Read the model definition and answer for the solid it produces. Units are mm, in the model's axes. A direction names the side the tool comes from. Give positions to 0.01 mm unless a question says otherwise; leave off trailing zeros. Order: outer loops, then holes, each group sorted by start corner. A loop starts at its lowest first (then second) coordinate and runs counter-clockwise, first axis right, second up.
```python
from build123d import *

# Parameters (mm, degrees)
EXTRUDE_1_DEPTH = 3
CHAMFER_1_SIZE  = 0.3065
CHAMFER_2_SIZE  = 0.5
FILLET_1_R      = 0.3


with BuildPart() as part:
    # 草圖1 → 填料-伸長1 (new body)
    with BuildSketch(Plane(origin=(-3, 0, 0), x_dir=(0, -1, 0), z_dir=(-1, 0, 0))):
        with BuildLine():
            Line((2.449489743, 2.5), (-2.449489743, 2.5))
            ThreePointArc((-2.449489743, 2.5), (-3.5, 0), (-2.449489743, -2.5))
            Line((-2.449489743, -2.5), (2.449489743, -2.5))
            ThreePointArc((2.449489743, -2.5), (3.5, 0), (2.449489743, 2.5))
        make_face()
    extrude(amount=-EXTRUDE_1_DEPTH)

    # 草圖2 → 旋轉1 (revolve)
    with BuildSketch(Plane.XY, mode=Mode.PRIVATE) as revolve_1_sk:
        Polygon((0, 1.95), (0, 0), (11, 0), (11, 1.5), (6.2, 1.5), (6.2, 1.05), (5, 1.05), (5, 2), (1.5, 2), (1.5, 1.95), align=None)
    revolve(revolve_1_sk.sketch.rotate(Axis((0, 0, 0), (1, 0, 0)), 270), axis=Axis((0, 0, 0), (1, 0, 0)))

    # 導角1
    chamfer_1_edges = [part.edges().sort_by_distance(p)[0] for p in [
        (11, 0, 1.5),
    ]]
    chamfer(chamfer_1_edges, length=CHAMFER_1_SIZE)

    # 導角2
    chamfer_2_edges = [part.edges().sort_by_distance(p)[0] for p in [
        (-3, 3.5, 0),
        (-3, -3.5, 0),
    ]]
    chamfer(chamfer_2_edges, length=CHAMFER_2_SIZE)

    # 圓角1
    fillet_1_edges = [part.edges().sort_by_distance(p)[0] for p in [
        (6.2, 0, 1.05),
        (5, 0, 1.05),
    ]]
    fillet(fillet_1_edges, radius=FILLET_1_R)


solid = part.part
```
1) The part is cut by section A-A on z = 0. Determine the outline of the cut face in (x, y), and give its area (3 significant figures).
Final values:
outline: (-3, -3) - (-2.5, -3.5) - (0, -3.5) - (0, -1.95) - (1.5, -1.95) - (1.5, -2) - (5, -2) - (5, -1.35) arc R0.3 cw to (5.3, -1.05) - (5.9, -1.05) arc R0.3 cw to (6.2, -1.35) - (6.2, -1.5) - (10.69, -1.5) - (11, -1.19) - (11, 1.19) - (10.69, 1.5) - (6.2, 1.5) - (6.2, 1.35) arc R0.3 cw to (5.9, 1.05) - (5.3, 1.05) arc R0.3 cw to (5, 1.35) - (5, 2) - (1.5, 2) - (1.5, 1.95) - (0, 1.95) - (0, 3.5) - (-2.5, 3.5) - (-3, 3) - close
area: 57.5 mm2
2) The part is cut by section B-B on y = 0. Determine the outline of the cut face in (x, z), and give its area (3 significant figures).
Final values:
outline: (-3, -2.5) - (0, -2.5) - (0, -1.95) - (1.5, -1.95) - (1.5, -2) - (5, -2) - (5, -1.35) arc R0.3 cw to (5.3, -1.05) - (5.9, -1.05) arc R0.3 cw to (6.2, -1.35) - (6.2, -1.5) - (10.69, -1.5) - (11, -1.19) - (11, 1.19) - (10.69, 1.5) - (6.2, 1.5) - (6.2, 1.35) arc R0.3 cw to (5.9, 1.05) - (5.3, 1.05) arc R0.3 cw to (5, 1.35) - (5, 2) - (1.5, 2) - (1.5, 1.95) - (0, 1.95) - (0, 2.5) - (-3, 2.5) - close
area: 51.8 mm2
3) Given pin 1 (3 mm diameter, centred on y = 2, z = 0, fed in from +X), flat-ended and moving along its own axis, determine where the tip first touches the part or whether it passes through.
Final values:
pin 1: stops at x = 11
4) The part is cut by section D-D on x = 8.75. Determine the outline of the cut face in (y, z).
Final values:
outline: circle Ø3 at (0, 0)
5) A tool of negligible diameter and unlimited length cuts with its end or side. For faces 5 (the face through (5.6, 0.32, -1)), 6 (the face through (-1.3, 3.5, 0)), 7 (the face through (8.42, 0.45, -1.43)), from which of +Z, -Z, +X, -X, +Y, -Y can it reach the whole face along a straight path? Write none if from no direction.
Final values:
face 5: none
face 6: +X, -X, +Y
face 7: +X
6) The part is cut by section C-C on x = 1. Determine the outline of the cut face in (y, z), and give its area (3 significant figures).
Final values:
outline: circle Ø3.9 at (0, 0)
area: 11.9 mm2
7) For a pull along X with two mould halves and no side action, classify faces 1 (the face through (-3, 0, 0)), 2 (the face through (0.74, -1.187, 1.547)), 3 (the face through (11, 0, 0)), 4 (the face through (-1.3, -3.5, 0)) as released by +X, released by -X, zero draft, split by the parting line, or undercut.
Final values:
face 1: released by -X
face 2: undercut
face 3: released by +X
face 4: zero draft
8) Consider L1, parallel to X at y = 1.25, z = 0.1; L2, parallel to X at y = -2.5, z = 0; L3, parallel to Y at x = 10, z = 0.95. Determine where each line is inside the solid, lowest interval first.
Final values:
L1: x = -3 to 5.02, 6.18 to 10.94
L2: x = -3 to 0
L3: y = -1.16 to 1.16
